The listing builds one solid part. Answer for the finished solid, in the listing's coordinates (mm). A direction names the side the tool comes from. Coordinates: 2 decimals unless noted, no trailing zeros. Write each loop counter-clockwise with the first axis right and the second up, starting at its lowest first coordinate (ties: lowest second). Pieces come first, ordered by that corner, then holes.
(1) Given P1, Ø1.5, axis at x = 1.5, y = 4.5, coming from the -Z side; P2, Ø2, axis at x = 1, z = -0.5, coming from the -Y side, each flat-ended and moving along its own axis, determine where each tip first touches the part or whether it passes through.
(2) The part is cut by section A-A on y = 0. Determine the outline of the cut face in (x, z), plus the area to 3 significant figures.
(3) The part is cut by section C-C on x = -1.15. Determine the outline of the cut face in (y, z).
(4) Which of the six approach directions +Z, -Z, +X, -X, +Y, -Y give full straight-line access (tool end or side, diameter ignored) to faces 1 (the flat face through (1, -4, 4)), 2 (the cylindrical face through (-0.03, -1.5, -0.07))?
(5) Straight lines are drawn through the part: line 1 (X direction, y = -1.5, z = 5.5); line 2 (Z direction, x = -0.25, y = 0); line 3 (Z direction, x = 1.45, y = 0). For each, find the intervals that lie inside material, in ascending order.
(6) The part is cut by section D-D on z = -3.5. Determine the outline of the cut face in (x, y), plus the area to 3 significant figures.
(7) For a pull along X with two mould halves and no side action, classify faces 3 (the cylindrical face through (1.507, -5.994, 0.264)), 4 (the flat face through (-1, -4, 4)), 5 (the flat face through (-2, 1.2, -1.2)) as +X half, -X half, draft (parallel to the pull), parting line (faces both ways), or undercut.
Autodesk Inventor part; units mm, degrees
ref_plane "YZ Plane" through (0, 0, 0) normal (1, 0, 0) x (0, 1, 0)
ref_plane "XZ Plane" through (0, 0, 0) normal (0, 1, 0) x (-1, 0, 0)
ref_plane "XY Plane" through (0, 0, 0) normal (0, 0, 1) x (1, 0, 0)
sketch "スケッチ1" plane through (0, 0, 0) normal (0, 0, 1) x (1, 0, 0)
  line L0 (-2, 6) -> (-1, 6)
  line L1 (-1, 6) -> (-1, 5)
  line L2 (-1, 5) -> (1, 5)
  line L3 (1, 5) -> (1, 6)
  line L4 (1, 6) -> (2, 6)
  line L5 (2, 6) -> (2, 1.5)
  line L6 (2, 1.5) -> (-2, 1.5)
  line L7 (-2, 1.5) -> (-2, 6)
  line L8 (0, -1.2) -> (0, 7.2) construction
  line L9 (-2.8, 0) -> (2.8, 0)
  point P0 (0, 0)
  dimension "d0" = 1.5
  dimension "d1" = 5
  dimension "d2" = 1
  dimension "d3" = 2
  dimension "d4" = 1
revolve "回転1" add sketch "スケッチ1" angle 360 about axis through (-10, 0, 0) along (1, 0, 0)
properties part number "Pulley_L"
Model answer:
1. P1: stops at z = -4.68
1. P2: stops at y = -6
2. outline: (-2, -6) - (-1, -6) - (-1, -5) - (1, -5) - (1, -6) - (2, -6) - (2, -1.5) - (-2, -1.5) - close; (-2, 1.5) - (2, 1.5) - (2, 6) - (1, 6) - (1, 5) - (-1, 5) - (-1, 6) - (-2, 6) - close
2. area: 32.0 mm2
3. outline: circle Ø12 at (0, 0); hole circle Ø3 at (0, 0)
4. face 1: none
4. face 2: +X, -X
5. line 1: x = -2 to -1, 1 to 2
5. line 2: z = -5 to -1.5, 1.5 to 5
5. line 3: z = -6 to -1.5, 1.5 to 6
6. outline: (-2, -4.87) - (-1, -4.87) - (-1, -3.57) - (1, -3.57) - (1, -4.87) - (2, -4.87) - (2, 4.87) - (1, 4.87) - (1, 3.57) - (-1, 3.57) - (-1, 4.87) - (-2, 4.87) - close
6. area: 33.8 mm2
7. face 3: draft
7. face 4: undercut
7. face 5: -X half
